from build123d import *

# Parameters (mm, degrees)
SKETCH2_R           = 5
SKETCH2_R_2         = 2.5
BOSS_EXTRUDE1_DEPTH = 2
SKETCH2_3_R         = 2.5
BOSS_EXTRUDE2_DEPTH = 25
CUT_EXTRUDE1_START  = -25
SKETCH3_R           = 1.5
CUT_EXTRUDE1_DEPTH  = 53.910571474


with BuildPart() as part:
    # Sketch2 → Boss-Extrude1 (new body)
    # profile 1 of 2: a face of its own
    with BuildSketch(Plane(origin=(0, 0, 0), x_dir=(1, 0, 0), z_dir=(0, 1, 0))):
        with Locations(Location((0, 0, 0), (0, 0, 270))):
            Circle(SKETCH2_R)
        Circle(SKETCH2_R_2, mode=Mode.SUBTRACT)
    # profile 2 of 2: a face of its own
    with BuildSketch(Plane(origin=(0, 0, 0), x_dir=(1, 0, 0), z_dir=(0, 1, 0))):
        Circle(SKETCH2_R_2)
    extrude(amount=-BOSS_EXTRUDE1_DEPTH)

    # Sketch2<3> → Boss-Extrude2 (add)
    with BuildSketch(Plane(origin=(0, 0, 0), x_dir=(1, 0, 0), z_dir=(0, 1, 0))):
        with Locations(Location((0, 0, 0), (0, 0, 270))):
            Circle(SKETCH2_3_R)
    extrude(amount=BOSS_EXTRUDE2_DEPTH)

    # Sketch3 → Cut-Extrude1 (cut, through all)
    with BuildSketch(Plane(origin=(0, 25, 0), x_dir=(1, 0, 0), z_dir=(0, 1, 0)).offset(CUT_EXTRUDE1_START)):
        with Locations(Location((0, 0, 0), (0, 0, 270))):
            Circle(SKETCH3_R)
    extrude(amount=CUT_EXTRUDE1_DEPTH, mode=Mode.SUBTRACT)


solid = part.part
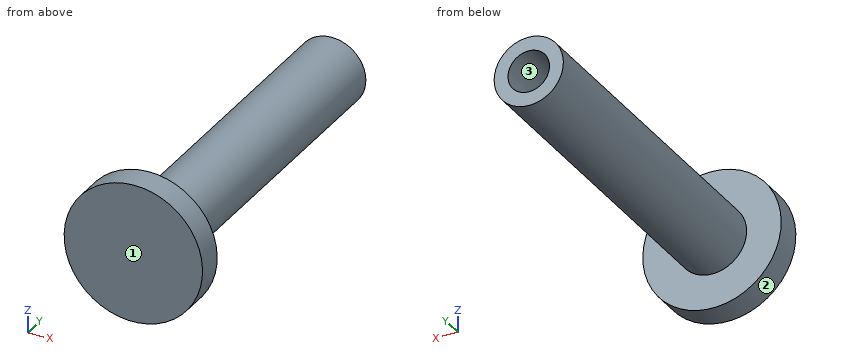
Could you check a few things on this model? Use its own coordinates, in mm. Face numbers are marked on the shaded views. Give positions to 0.01 mm unless a question says otherwise; leave off trailing zeros. Order: outer loops, then holes, each group sorted by start corner. A loop starts at its lowest first (then second) coordinate and runs counter-clockwise, first axis right, second up. Notation, with made-up numbers: (83.25, -22.5) - (89.25, -22.5) arc R24 cw to (89.25, 4.5) - close; hole circle Ø9 at (6, -32.75). An arc over 180 degrees is marked (long way). One line per item, written item: value. Start each with the question number.
1. Thinking about a two-plate mould opening in Z: for the marked faces 1, 2 and 3, which applies, +Z half, -Z half, draft (parallel to the pull), parting line (faces both ways), or undercut?
2. Imagine slicing it at A-A on x = 0. List the corners of the cut face in (y, z) for me, plus the area to 3 significant figures.
3. Imagine slicing it at C-C on z = 0. List the corners of the cut face in (x, y) for me, plus the area to 3 significant figures.
4. For P1, Ø6, axis at x = 3, y = 18, coming from the -Z side; P2, Ø3, axis at y = 5, z = -2.5, coming from the +X side; P3, Ø1.5, axis at x = 0.5, z = 0, coming from the +Y side, each with a flat end and sliding along its axis, tell me the tip position at first contact or that it passes through.
5. Imagine slicing it at B-B on y = 11.75. List the corners of the cut face in (x, z) for me.
6. Imagine slicing it at D-D on z = 4. List the corners of the cut face in (x, y) for me.
7. If I drill on probe 1 along X at (y, z) = (9.5, 0); probe 2 along Y at (x, z) = (0.5, 3); probe 3 along X at (y, z) = (19.75, -1), over which ranges is the centre line in solid material (lowest first)?
Values:
1. face 1: draft
1. face 2: parting line
1. face 3: undercut
2. outline: (-2, -5) - (0, -5) - (0, -2.5) - (25, -2.5) - (25, -1.5) - (0, -1.5) - (0, 1.5) - (25, 1.5) - (25, 2.5) - (0, 2.5) - (0, 5) - (-2, 5) - close
2. area: 70.0 mm²
3. outline: (-5, -2) - (5, -2) - (5, 0) - (2.5, 0) - (2.5, 25) - (1.5, 25) - (1.5, 0) - (-1.5, 0) - (-1.5, 25) - (-2.5, 25) - (-2.5, 0) - (-5, 0) - close
3. area: 70.0 mm²
4. P1: z = -2.5
4. P2: x = 2.29
4. P3: y = 0
5. outline: circle Ø5 at (0, 0); hole circle Ø3 at (0, 0)
6. outline: (-3, -2) - (3, -2) - (3, 0) - (-3, 0) - close
7. probe 1: -2.5 to -1.5, 1.5 to 2.5
7. probe 2: -2 to 0
7. probe 3: -2.29 to -1.12, 1.12 to 2.29
